Drawing for the job (mm, zero at the part's lowest x, y, z). A direction names the side the tool comes from. Coordinates: 2 decimals unless noted, no trailing zeros. Loops run counter-clockwise (first coordinate to the right, second up) from the corner with the lowest first, then second, coordinate; pieces in that order, holes last. Notation, with made-up numbers: (-24.5, 84) - (17.5, 84) arc R21 ccw to (17.5, 120) - close; hole circle Ø8 at (-33.75, -28.75). An arc over 180 degrees is marked (long way). One line per item, written item: value.
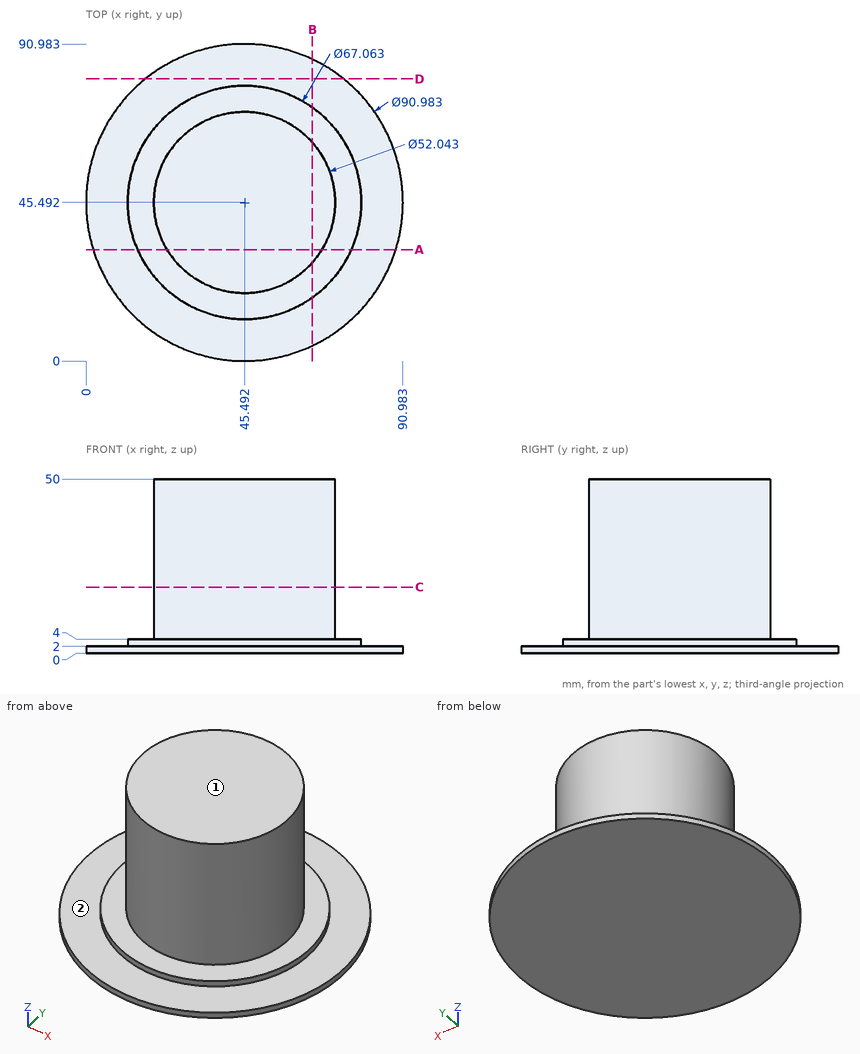
Item 1: Cut at D-D, the plane y = 81. Write the cut outline in (x, z) (1 decimal).
Check result:
outline: (17.1, 0) - (73.9, 0) - (73.9, 2) - (17.1, 2) - close
Item 2: Drop flat-ended pins along their axis: P1, Ø8, axis at x = 61, z = 17.5, coming from the -Y side; P2, Ø1, axis at x = 16.5, y = 52, coming from the +Z side; P3, Ø5, axis at x = 19.5, y = 79.5, coming from the +Z side. Give the stop position or say it passes through.
Check result:
P1: stops at y = 22.15
P2: stops at z = 4
P3: stops at z = 2
Item 3: Probe probe 1 along Z at (x, y) = (73, 54); probe 2 along Z at (x, y) = (67.5, 85); probe 3 along Y at (x, z) = (43.5, 27.5). List the from-to ranges inside material, lowest first. Write a range as from..to.
Check result:
probe 1: z = 0..4
probe 2: z = 0..2
probe 3: y = 19.55..71.44
Item 4: Tool access for the marked faces 1 and 2: list every direction of +Z, -Z, +X, -X, +Y, -Y with a clear straight run to the whole face (end or side of a thin tool).
Check result:
face 1: +Z, +X, -X, +Y, -Y
face 2: +Z
Item 5: Cut at B-B, the plane x = 65. Write the cut outline in (y, z) (1 decimal), then the cut area to 3 significant figures.
Check result:
outline: (4.4, 0) - (86.6, 0) - (86.6, 2) - (72.8, 2) - (72.8, 4) - (62.7, 4) - (62.7, 50) - (28.3, 50) - (28.3, 4) - (18.2, 4) - (18.2, 2) - (4.4, 2) - close
area: 1,860 mm^2
Item 6: Cut at A-A, the plane y = 32. Write the cut outline in (x, z) (1 decimal), then the cut area to 3 significant figures.
Check result:
outline: (2, 0) - (88.9, 0) - (88.9, 2) - (76.2, 2) - (76.2, 4) - (67.7, 4) - (67.7, 50) - (23.2, 50) - (23.2, 4) - (14.8, 4) - (14.8, 2) - (2, 2) - close
area: 2,340 mm^2
Item 7: Cut at C-C, the plane z = 19. Write the cut outline in (x, y), then the cut area to 3 significant figures.
Check result:
outline: circle Ø52.04 at (45.49, 45.49)
area: 2,130 mm^2
